```python
from build123d import *

# Parameters (mm, degrees)
F1_DEPTH    = 2
F2_T1_DEPTH = 2
F2_T3_DEPTH = 2.7234665539
F2_T5_DEPTH = 4.5


# Not quite as in the source:
# - a fillet or chamfer that OpenCascade refuses, or shapes differently, is made with other operations: its cross-section is extruded or revolved along the edge and cut away or added


with BuildPart() as f1:
    # F0 (on Top) → F1 (new body)
    with BuildSketch(Plane.XY):
        Polygon((0, 0.7), (0, 0), (30, 0), (30, 0.7), (2.4998066677, 0.7), (5.0013818819, 4.6602413969), (4.5786552685, 4.9272661341), (1.9084078958, 0.7), (1.0515667407, 1.2412429146), (3.7218141134, 5.4685090487), (3.2145421773, 5.7889387335), align=None)
    extrude(amount=F1_DEPTH)

    # F2: fillet of radius 0.5 on 4 edges, made by hand

    # F2_s2 → F2_t1 (join)
    with BuildSketch(Plane.XY):
        with BuildLine():
            ThreePointArc((3.4070416429, 0.7), (2.9691419006, 0.9586624445), (2.9843150295, 1.4670247373))
            Line((2.9843150295, 1.4670247373), (2.4998066677, 0.7))
            Line((2.4998066677, 0.7), (3.4070416429, 0.7))
        make_face()
    extrude(amount=F2_T1_DEPTH)

    # F2_s4 → F2_t3 (cut)
    with BuildSketch(Plane.XY.offset(-0.3617332769)):
        with BuildLine():
            ThreePointArc((0.0772733866, 0.8223314265), (0.0197067007, 0.6942971445), (0, 0.5553066892))
            Line((0, 0.5553066892), (0, 0.7))
            Line((0, 0.7), (0.0772733866, 0.8223314265))
        make_face()
    extrude(amount=F2_T3_DEPTH, mode=Mode.SUBTRACT)

    # F2_s6 → F2_t5 (cut)
    with BuildSketch(Plane.XY.offset(-1.25)):
        with BuildLine():
            ThreePointArc((3.6372687907, 5.5219139962), (3.2601462009, 5.5869152402), (2.94751744, 5.3662121201))
            Line((2.94751744, 5.3662121201), (3.2145421773, 5.7889387335))
            Line((3.2145421773, 5.7889387335), (3.6372687907, 5.5219139962))
        make_face()
        with BuildLine():
            ThreePointArc((3.4547893761, 5.0457824353), (3.5197906201, 5.4229050251), (3.2990874999, 5.735533786))
            Line((3.2990874999, 5.735533786), (3.7218141134, 5.4685090487))
            Line((3.7218141134, 5.4685090487), (3.4547893761, 5.0457824353))
        make_face()
    extrude(amount=F2_T5_DEPTH, mode=Mode.SUBTRACT)


solid = f1.part
```
Input: part model. Units: mm. Frame: model coordinates. A direction names the side the tool comes from. Round coordinates to 2 decimals unless told otherwise and drop trailing zeros. Loops run counter-clockwise (first coordinate to the right, second up) from the corner with the lowest first, then second, coordinate; pieces in that order, holes last. Notation, with made-up numbers: (-32.75, 70) -> (11.25, 70) arc R8 ccw to (11.25, 80) -> close; hole circle Ø5 at (89.5, 28.25). An arc over 180 degrees is marked (long way). One line per item, written item: value.
(1) Section D-D (x = 15.5). Return the cut outline in (y, z).
Geometry check:
outline: (0, 0) -> (0.7, 0) -> (0.7, 2) -> (0, 2) -> close
(2) Section B-B (y = 3.25). Return the cut outline in (x, z).
Geometry check:
outline: (1.61, 0) -> (2.32, 0) -> (2.32, 2) -> (1.61, 2) -> close; (3.52, 0) -> (4.11, 0) -> (4.11, 2) -> (3.52, 2) -> close
(3) Set-up query: faces 1 (the face through (2.24, 3.12, 0.99)), 2 (the face through (11.6, 0.5, 2)), 3 (the face through (3.98, 3.04, 0.99)). Return all of +Z, -Z, +X, -X, +Y, -Y with unobstructed straight access to the full face (end or side cutting, diameter ignored); none if empty.
Geometry check:
face 1: +Z, -Z
face 2: +Z, +X, -X, +Y, -Y
face 3: +Z, -Z, +X
(4) Material intervals for line 1 (Y direction, x = 3.25, z = 1.3); line 2 (Y direction, x = 22, z = 0.25); line 3 (X direction, y = 4.45, z = 1.5), sorted ascending. Write a range as [from, to].
Geometry check:
line 1: [0, 0.73], [1.89, 2.82], [4.72, 5.58]
line 2: [0, 0.7]
line 3: [2.37, 3.08], [4.28, 4.87]
(5) Section C-C (z = 0.7). Return the cut outline in (x, y).
Geometry check:
outline: (0, 0) -> (30, 0) -> (30, 0.7) -> (3.41, 0.7) arc R0.5 cw to (2.98, 1.47) -> (5, 4.66) -> (4.58, 4.93) -> (1.91, 0.7) -> (1.05, 1.24) -> (3.45, 5.05) arc R0.5 ccw to (3.45, 5.59) arc R0.5 ccw to (2.95, 5.37) -> (0.08, 0.82) arc R0.5 ccw to (0, 0.56) -> close
(6) Section A-A (x = 2.5). Return the cut outline in (y, z), plus the area to 3 significant figures.
Geometry check:
outline: (0, 0) -> (1.64, 0) -> (1.64, 2) -> (0, 2) -> close; (3.53, 0) -> (4.66, 0) -> (4.66, 2) -> (3.53, 2) -> close
area: 5.52 mm2
(7) Mould query, pull axis Y, two halves, no side actions, for faces 4 (the face through (3.26, 2.84, 0.99)), 5 (the face through (15, 0, 1)), 6 (the face through (1.532, 3.126, 0.986)), 7 (the face through (11.6, 0.5, 0)). Classes: pulls with the +Y half, pulls with the -Y half, needs draft (parallel to the pull), parting line crosses it, or undercut.
Geometry check:
face 4: undercut
face 5: pulls with the -Y half
face 6: pulls with the +Y half
face 7: needs draft
